from build123d import *
from build123d import SkipClean  # not in build123d's __all__

# Parameters (mm, degrees)
F0_R     = 2.5
F1_DEPTH = 1
F2_DEPTH = 3
F0_R_2   = 1
F3_DEPTH = 1


# Not quite as in the source:
# - after a boolean that leaves OpenCascade's solid faulty, fix() repairs it


with BuildPart() as f1:
    # F0 (on Top) → F1 (new body)
    with BuildSketch(Plane.XY):
        with BuildLine():
            ThreePointArc((-12.5, 0), (-13.1609318732, 1.4855627054), (-14.7068965517, 1.9892696692))
            ThreePointArc((-14.7068965517, 1.9892696692), (-16.5, 0), (-14.7068965517, -1.9892696692))
            ThreePointArc((-14.7068965517, -1.9892696692), (-13.1609318732, -1.4855627054), (-12.5, 0))
        make_face()
        with BuildLine():
            ThreePointArc((-0.362068922, -3.4812219257), (-3.5, 7.5e-09), (-0.362068907, 3.4812219272))
            Line((-0.362068907, 3.4812219272), (-14.7068965517, 1.9892696692))
            ThreePointArc((-14.7068965517, 1.9892696692), (-13.1609318732, 1.4855627054), (-12.5, 0))
            ThreePointArc((-12.5, 0), (-13.1609318732, -1.4855627054), (-14.7068965517, -1.9892696692))
            Line((-14.7068965517, -1.9892696692), (-0.362068922, -3.4812219257))
        make_face()
        with BuildLine():
            ThreePointArc((-0.362068922, -3.4812219257), (2.3433692382, -2.5997347198), (3.5, 0))
            ThreePointArc((3.5, 0), (2.3433692438, 2.5997347148), (-0.362068907, 3.4812219272))
            ThreePointArc((-0.362068907, 3.4812219272), (-3.5, 7.5e-09), (-0.362068922, -3.4812219257))
        make_face()
        Circle(F0_R, mode=Mode.SUBTRACT)
    extrude(amount=F1_DEPTH)

    # F0 (on Top) → F2 (join)
    with BuildSketch(Plane.XY):
        with BuildLine():
            ThreePointArc((-0.362068922, -3.4812219257), (2.3433692382, -2.5997347198), (3.5, 0))
            ThreePointArc((3.5, 0), (2.3433692438, 2.5997347148), (-0.362068907, 3.4812219272))
            ThreePointArc((-0.362068907, 3.4812219272), (-3.5, 7.5e-09), (-0.362068922, -3.4812219257))
        make_face()
        Circle(F0_R, mode=Mode.SUBTRACT)
    with SkipClean():  # cleaning this boolean's faces spoils the solid; the shape is the same uncleaned
        extrude(amount=-F2_DEPTH)

    # F0 (on Top) → F3 (join)
    with BuildSketch(Plane.XY):
        Circle(F0_R)
        Circle(F0_R_2, mode=Mode.SUBTRACT)
    extrude(amount=-F3_DEPTH)

    add(f1.part.fix(), mode=Mode.REPLACE)


solid = f1.part
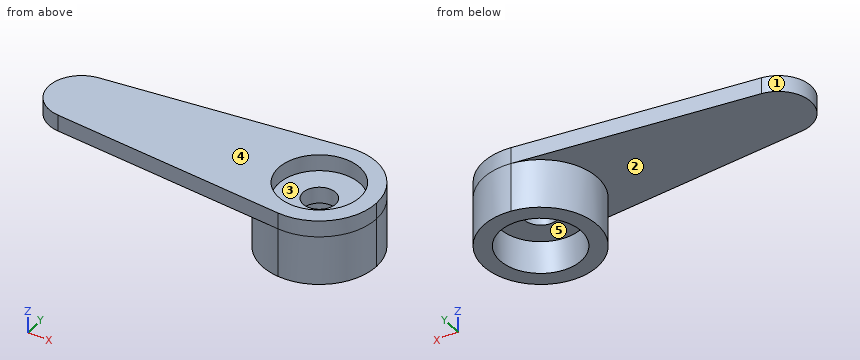
Geometry check sheet. Reference: the model listing, model coordinates, mm. Face numbers are marked on the shaded views. A direction names the side the tool comes from. Give positions to 0.01 mm unless a question says otherwise; leave off trailing zeros. Order: outer loops, then holes, each group sorted by start corner. A loop starts at its lowest first (then second) coordinate and runs counter-clockwise, first axis right, second up.
1) Cross-section at A-A (x = 0). Record the boundary of the cut face in (y, z).
Results are:
outline: (-3.5, -3) - (-2.5, -3) - (-2.5, -1) - (-1, -1) - (-1, 0) - (-2.5, 0) - (-2.5, 1) - (-3.5, 1) - close; (1, -1) - (2.5, -1) - (2.5, -3) - (3.5, -3) - (3.5, 1) - (2.5, 1) - (2.5, 0) - (1, 0) - close
2) Cross-section at B-B (y = -0.5). Record the boundary of the cut face in (x, z), then the cut area to 3 significant figures.
Results are:
outline: (-16.44, 0) - (-3.46, 0) - (-3.46, -3) - (-2.45, -3) - (-2.45, -1) - (-0.87, -1) - (-0.87, 0) - (-2.45, 0) - (-2.45, 1) - (-16.44, 1) - close; (0.87, -1) - (2.45, -1) - (2.45, -3) - (3.46, -3) - (3.46, 1) - (2.45, 1) - (2.45, 0) - (0.87, 0) - close
area: 24.3 mm2
3) Draft check along Y on the marked faces 1, 2 and 3. Enter one of: released by +Y, released by -Y, zero draft, split by the parting line, or undercut.
Results are:
face 1: split by the parting line
face 2: zero draft
face 3: undercut
4) Cross-section at C-C (z = -2.7). Record the boundary of the cut face in (x, y).
Results are:
outline: circle Ø7 at (0, 0); hole circle Ø5 at (0, 0)
5) Gauge pin test, flat ends, axial feed: pin 1 (1 mm diameter, centred on y = -0.5, z = 0.5, fed in from -X); pin 2 (3 mm diameter, centred on x = 0, y = 0, fed in from +Z). Record the tip position at first contact, or that the pin passes through.
Results are:
pin 1: stops at x = -16.5
pin 2: stops at z = 0
6) Cross-section at D-D (y = -3). Record the boundary of the cut face in (x, z).
Results are:
outline: (-4.99, 0) - (-1.8, 0) - (-1.8, -3) - (1.8, -3) - (1.8, 1) - (-4.99, 1) - close
7) Tool access check on the marked faces 4 and 5. Record the directions out of +Z, -Z, +X, -X, +Y, -Y that give a thin tool (end or side, any length) a straight path to the whole face; none if there is none.
Results are:
face 4: +Z, +X, -X, +Y, -Y
face 5: -Z
8) Material ranges on probe 1 along Y at (x, z) = (0, 0.6); probe 2 along Z at (x, y) = (-8.75, -1); probe 3 along Z at (x, y) = (1, 0.25), recorded low to high.
Results are:
probe 1: y = -3.5 to -2.5, 2.5 to 3.5
probe 2: z = 0 to 1
probe 3: z = -1 to 0
